The model under review builds one solid part; all positions refer to its coordinate system, in mm. A direction names the side the tool comes from. Give positions to 0.01 mm unless a question says otherwise; leave off trailing zeros. Order: outer loops, then holes, each group sorted by start corner. A loop starts at its lowest first (then second) coordinate and runs counter-clockwise, first axis right, second up. Notation, with made-up numbers: (2, 64) - (20, 64) arc R15 ccw to (20, 76) - close; hole circle Ø8 at (5.5, 72). An arc over 180 degrees is marked (long way). Use CSV: the item, a comma, the result in double quotes. Start each with the question number.
1. To check wall thickness, follow line 1 (X direction, y = 22, z = 1.95); line 2 (Y direction, x = 44, z = 2.5). State the ranges of each line that lie inside material, in increasing order. Write a range as [from, to].
2. For pin 1 (1.2 mm diameter, centred on x = 28.5, z = 2.5, fed in from +Y); pin 2 (10 mm diameter, centred on x = 26.5, y = 26, fed in from -Z); pin 3 (1.2 mm diameter, centred on y = 16, z = 2.5, fed in from -X); pin 4 (0.8 mm diameter, centred on y = 13.5, z = 2, fed in from +X), all flat-tipped, find the tip position at first contact; note any pin that passes through.
3. Take a section at B-B, the plane y = 22. State the section outline as (x, z) points.
4. Take a section at A-A, the plane x = 38.5. State the section outline as (y, z) points.
5. Machinability: for faces 1 (the flat face through (26, 3, 2)), 2 (the cylindrical face through (47.669, 38.686, 2.26)), 3 (the cylindrical face through (3.314, 38.669, 2.26)), 4 (the cylindrical face through (3.331, 3.314, 2.26)), 5 (the cylindrical face through (47.686, 3.331, 2.26)), which of the approach directions +Z, -Z, +X, -X, +Y, -Y give a long, thin tool a straight path to every point of the face, cutting with its end or side? Answer none if there is none.
```python
from build123d import *

# Parameters (mm, degrees)
EXTRUDE_1_DEPTH     = 3
SKETCH_2_OUTSIDE_W  = 66.228
SKETCH_2_OUTSIDE_H  = 57.228
CUT_EXTRUDE_1_DEPTH = 1.5


with BuildPart() as part:
    # 草图1 → 凸台-拉伸1 (new body)
    with BuildSketch(Plane.XY):
        with BuildLine():
            Line((3, 0), (48, 0))
            ThreePointArc((48, 0), (50.121320344, 0.878679656), (51, 3))
            Line((51, 3), (51, 39))
            ThreePointArc((51, 39), (50.121320344, 41.121320344), (48, 42))
            Line((48, 42), (3, 42))
            ThreePointArc((3, 42), (0.878679656, 41.121320344), (0, 39))
            Line((0, 39), (0, 3))
            ThreePointArc((0, 3), (0.878679656, 0.878679656), (3, 0))
        make_face()
    extrude(amount=EXTRUDE_1_DEPTH)

    # 草图2 outside → 切除-拉伸1 (cut)
    with BuildSketch(Plane.XY.offset(3)):
        with Locations((25.5, 21)):
            Rectangle(SKETCH_2_OUTSIDE_W, SKETCH_2_OUTSIDE_H)
        with BuildLine():
            Line((4.1, 39), (46.9, 39))
            ThreePointArc((46.9, 39), (47.677817459, 38.677817459), (48, 37.9))
            Line((48, 37.9), (48, 4.1))
            ThreePointArc((48, 4.1), (47.677817459, 3.322182541), (46.9, 3))
            Line((46.9, 3), (4.1, 3))
            ThreePointArc((4.1, 3), (3.322182541, 3.322182541), (3, 4.1))
            Line((3, 4.1), (3, 37.9))
            ThreePointArc((3, 37.9), (3.322182541, 38.677817459), (4.1, 39))
        make_face(mode=Mode.SUBTRACT)
    extrude(amount=-CUT_EXTRUDE_1_DEPTH, mode=Mode.SUBTRACT)


solid = part.part
```
Determined:
1,line 1,"x = [3, 48]"
1,line 2,"y = [3, 39]"
2,pin 1,"stops at y = 39"
2,pin 2,"stops at z = 0"
2,pin 3,"stops at x = 3"
2,pin 4,"stops at x = 48"
3,outline,"(0, 0) - (51, 0) - (51, 1.5) - (48, 1.5) - (48, 3) - (3, 3) - (3, 1.5) - (0, 1.5) - close"
4,outline,"(0, 0) - (42, 0) - (42, 1.5) - (39, 1.5) - (39, 3) - (3, 3) - (3, 1.5) - (0, 1.5) - close"
5,face 1,"+Z, +X, -X, -Y"
5,face 2,"+Z, +X, +Y"
5,face 3,"+Z, -X, +Y"
5,face 4,"+Z, -X, -Y"
5,face 5,"+Z, +X, -Y"
